Input: part model. Units: mm. Frame: model coordinates. A direction names the side the tool comes from. Coordinates: 2 decimals unless noted, no trailing zeros. Loops run counter-clockwise (first coordinate to the right, second up) from the corner with the lowest first, then second, coordinate; pieces in that order, holes last. Notation, with made-up numbers: M 84.25,-16.5 L 92.25,-16.5 A37 cw 92.25,19.5 Z; hole C -31.5,-16 d7. An arc over 180 degrees is marked long. Use a Markdown table: item, result. Add a question column.
1. Section B-B on z = 595. Output: boundary loops of the cut face in (x, y).
2. Section D-D on y = 90. Output: boundary loops of the cut face in (x, z).
3. Set-up query: faces 4 (the cylindrical face through (562.985, 1704.93, 556.847)), 5 (the cylindrical face through (696.056, 92.023, 640.956)), 6 (the flat face through (704, 91, 596)). Return all of +Z, -Z, +X, -X, +Y, -Y with unobstructed straight access to the full face (end or side cutting, diameter ignored); none if empty.
4. Section C-C on z = 399.5. Output: boundary loops of the cut face in (x, y).
5. Draft query along X for faces 1 (the flat face through (335, 854, 0)), 2 (the cylindrical face through (588.52, 1714.06, 637.92)), 3 (the flat face through (692, 128, 609)). Return one class per face: +X half, -X half, draft (parallel to the pull), parting line (faces both ways), or undercut.
6. Section A-A on y = 1536.5. Output: boundary loops of the cut face in (x, z), then the cut area to 3 significant figures.
7. Line query: L1, parallel to X at y = 545.5, z = 266.5; L2, parallel to Y at x = 521, z = 447.5; L3, parallel to Y at x = 671, z = 443. Output: solid intervals per line, ascending. Write a range as [from, to].
8. Pin query (flat end, axial travel): pin 1 (6 mm diameter, centred on y = 458, z = 476.5, fed in from +X); pin 2 (8 mm diameter, centred on x = 363, z = 334, fed in from +Y). Return the tip coordinate at first contact, or that it passes through.
```python
from build123d import *

# Parameters (mm, degrees)
CROQUIS1_W              = 680
CROQUIS1_H              = 1700
SALIENTE_EXTRUIR1_DEPTH = 700
REDONDEO1_R             = 15
CROQUIS4_R              = 40
SALIENTE_EXTRUIR4_DEPTH = 22
CROQUIS5_R              = 45
SALIENTE_EXTRUIR5_DEPTH = 12
REDONDEO3_R             = 4
CROQUIS6_R              = 40
SALIENTE_EXTRUIR6_DEPTH = 24
CROQUIS7_R              = 46
SALIENTE_EXTRUIR7_DEPTH = 12
REDONDEO5_R             = 4


with BuildPart() as part:
    # Croquis1 → Saliente-Extruir1 (new body)
    with BuildSketch(Plane.XY):
        with Locations((340, 850)):
            Rectangle(CROQUIS1_W, CROQUIS1_H)
    extrude(amount=SALIENTE_EXTRUIR1_DEPTH)

    # Redondeo1
    redondeo1_edges = [part.edges().sort_by_distance(p)[0] for p in [
        (680, 850, 700),
        (340, 1700, 700),
        (0, 850, 700),
        (340, 1700, 0),
        (680, 850, 0),
        (0, 850, 0),
        (0, 1700, 350),
        (680, 1700, 350),
    ]]
    fillet(redondeo1_edges, radius=REDONDEO1_R)

    # Croquis4 → Saliente-Extruir4 (add)
    with BuildSketch(Plane(origin=(0, 1700, 0), x_dir=(1, 0, 0), z_dir=(0, 1, 0))):
        with Locations(Location((575, -595, 0), (0, 0, 90))):
            Circle(CROQUIS4_R)
    extrude(amount=SALIENTE_EXTRUIR4_DEPTH)

    # Croquis5 → Saliente-Extruir5 (add)
    with BuildSketch(Plane(origin=(0, 1722, 0), x_dir=(1, 0, 0), z_dir=(0, 1, 0))):
        with Locations(Location((575, -595, 0), (0, 0, 270))):
            Circle(CROQUIS5_R)
    extrude(amount=-SALIENTE_EXTRUIR5_DEPTH)

    # Redondeo3
    redondeo3_edges = [part.edges().sort_by_distance(p)[0] for p in [
        (575, 1722, 550),
    ]]
    fillet(redondeo3_edges, radius=REDONDEO3_R)

    # Croquis6 → Saliente-Extruir6 (add)
    with BuildSketch(Plane(origin=(680, 0, 0), x_dir=(0, 0, -1), z_dir=(1, 0, 0))):
        with Locations(Location((-595, 90, 0), (0, 0, 180))):
            Circle(CROQUIS6_R)
    extrude(amount=SALIENTE_EXTRUIR6_DEPTH)

    # Croquis7 → Saliente-Extruir7 (add)
    with BuildSketch(Plane(origin=(704, 0, 0), x_dir=(0, 0, -1), z_dir=(1, 0, 0))):
        with Locations((-595, 90)):
            Circle(CROQUIS7_R)
    extrude(amount=-SALIENTE_EXTRUIR7_DEPTH)

    # Redondeo5
    redondeo5_edges = [part.edges().sort_by_distance(p)[0] for p in [
        (704, 90, 641),
    ]]
    fillet(redondeo5_edges, radius=REDONDEO5_R)


solid = part.part
```
Answers below:
| question | item | result |
|---|---|---|
| 1 | outline | M 0,0 L 680,0 L 680,50 L 692,50 L 692,44 L 700,44 A4 ccw 704,48 L 704,132 A4 ccw 700,136 L 692,136 L 692,130 L 680,130 L 680,1685 A15 ccw 665,1700 L 615,1700 L 615,1710 L 620,1710 L 620,1718 A4 ccw 616,1722 L 534,1722 A4 ccw 530,1718 L 530,1710 L 535,1710 L 535,1700 L 15,1700 A15 ccw 0,1685 Z |
| 2 | outline | M 0,15 A15 ccw 15,0 L 665,0 A15 ccw 680,15 L 680,555 L 692,555 L 692,549 L 700,549 A4 ccw 704,553 L 704,637 A4 ccw 700,641 L 692,641 L 692,635 L 680,635 L 680,685 A15 ccw 665,700 L 15,700 A15 ccw 0,685 Z |
| 3 | face 4 | none |
| 3 | face 5 | +X |
| 3 | face 6 | +Z, -Z, +X, +Y, -Y |
| 4 | outline | M 0,0 L 680,0 L 680,1685 A15 ccw 665,1700 L 15,1700 A15 ccw 0,1685 Z |
| 5 | face 1 | draft |
| 5 | face 2 | parting line |
| 5 | face 3 | undercut |
| 6 | outline | M 0,15 A15 ccw 15,0 L 665,0 A15 ccw 680,15 L 680,685 A15 ccw 665,700 L 15,700 A15 ccw 0,685 Z |
| 6 | area | 476,000 mm² |
| 7 | L1 | x = [0, 680] |
| 7 | L2 | y = [0, 1700] |
| 7 | L3 | y = [0, 1698.75] |
| 8 | pin 1 | stops at x = 680 |
| 8 | pin 2 | stops at y = 1700 |
